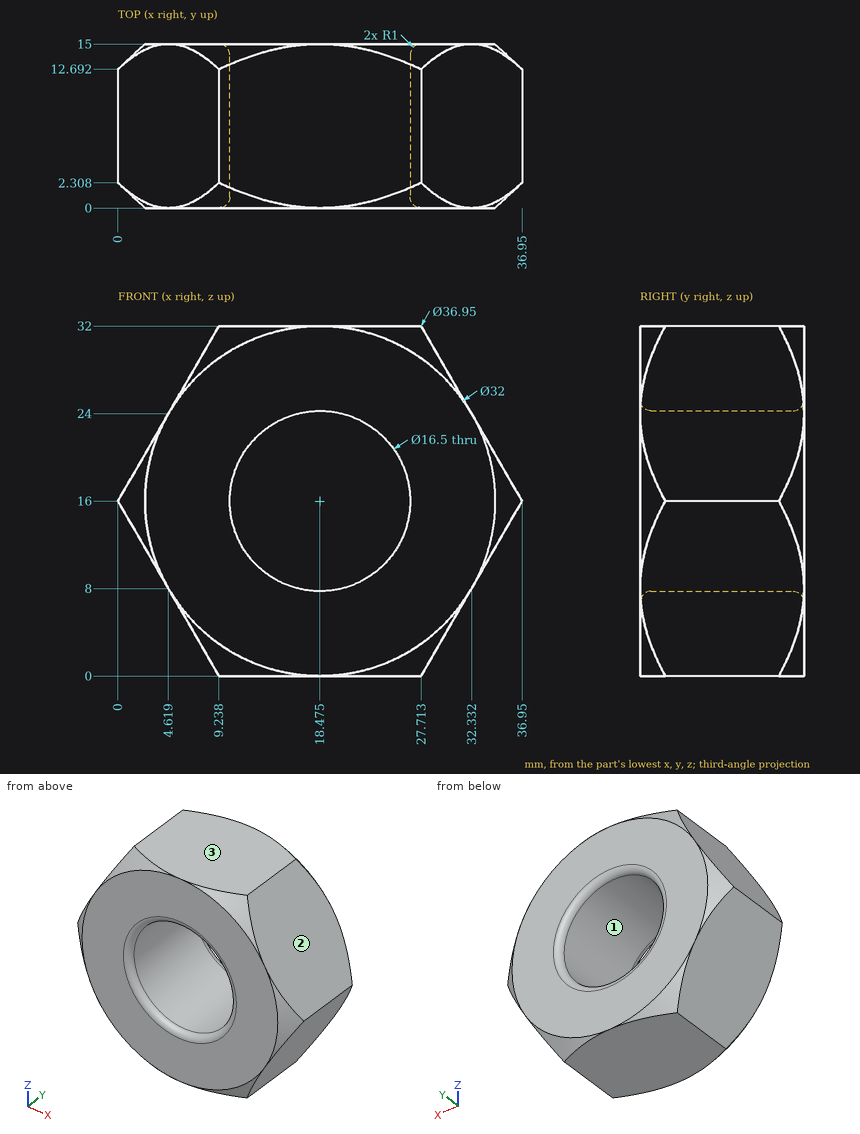
Design review of the part shown in the three views and the two pictorial views. Dimensions are in mm from the part's minimum x, y and z. Coordinates: 2 decimals unless noted, no trailing zeros.
Q1. To check wall thickness, follow line 1 (X direction, y = 2, z = 21) (1 decimal); line 2 (X direction, y = 5.25, z = 12); line 3 (Z direction, x = 24.5, y = 14.25) (1 decimal). State the ranges of each line that lie inside material, in increasing order.
Reported:
line 1: x = 2.9 to 11.9, 25 to 34.1
line 2: x = 2.31 to 11.26, 25.69 to 34.64
line 3: z = 0.3 to 10.3, 21.7 to 31.7
Q2. For pin 1 (1.5 mm diameter, centred on y = 5.5, z = 22.5, fed in from +X); pin 2 (8 mm diameter, centred on y = 11.5, z = 14.5, fed in from +X), all flat-tipped, find the tip position at first contact; note any pin that passes through.
Reported:
pin 1: stops at x = 33.63
pin 2: stops at x = 36.95
Q3. The part is to be moulded in two halves that separate along X. For the marked faces 1, 2 and 3, say which applies: +X half, -X half, draft (parallel to the pull), parting line (faces both ways), or undercut.
Reported:
face 1: undercut
face 2: +X half
face 3: draft
